from build123d import *

# Parameters (mm, degrees)
F1_DEPTH = 6.985
F2_R     = 5.08
F3_R     = 5.08
F4_R     = 1.27
F5_R     = 1.27


with BuildPart() as f1:
    # F0 (on Top) → F1 (new body)
    with BuildSketch(Plane.XY):
        with BuildLine():
            Line((13.4412104934, -0.1712630266), (10.8124273162, -2.0811858017))
            ThreePointArc((10.8124273162, -2.0811858017), (10.4719881953, -3.4025552234), (9.9707277708, -4.6716706359))
            Line((9.9707277708, -4.6716706359), (10.9748335954, -7.7619906019))
            ThreePointArc((10.9748335954, -7.7619906019), (18.0702175637, -8.5055805227), (23.2204469124, -13.442435522))
            Line((23.2204469124, -13.442435522), (27.3287873031, -8.8796612689))
            Line((27.3287873031, -8.8796612689), (26.6870015238, -2.7734774636))
            ThreePointArc((26.6870015238, -2.7734774636), (19.6185678945, -3.7402481997), (13.4412104934, -0.1712630266))
        make_face()
        with BuildLine():
            ThreePointArc((5.3205491095, 9.6401076749), (6.4720446345, 8.9080052234), (7.5241471277, 8.0391))
            Line((7.5241471277, 8.0391), (10.7735018328, 8.0391))
            ThreePointArc((10.7735018328, 8.0391), (13.6732921003, 14.5574292363), (19.960028611, 17.9300163252))
            Line((19.960028611, 17.9300163252), (16.8901194246, 23.2472550106))
            Line((16.8901194246, 23.2472550106), (10.8844708144, 24.5237950298))
            ThreePointArc((10.8844708144, 24.5237950298), (10.9792472078, 23.6942958469), (11.0109, 22.86))
            ThreePointArc((11.0109, 22.86), (9.1860721795, 16.789086006), (4.3164432849, 12.7304276409))
            Line((4.3164432849, 12.7304276409), (5.3205491095, 9.6401076749))
        make_face()
        with BuildLine():
            ThreePointArc((32.7520519625, 7.0641284914), (31.1139363339, 1.2856484198), (26.6870015238, -2.7734774636))
            Line((26.6870015238, -2.7734774636), (27.3287873031, -8.8796612689))
            Line((27.3287873031, -8.8796612689), (49.9321790072, 16.2239484353))
            Line((49.9321790072, 16.2239484353), (16.8901194246, 23.2472550106))
            Line((16.8901194246, 23.2472550106), (19.960028611, 17.9300163252))
            ThreePointArc((19.960028611, 17.9300163252), (28.869551071, 15.4561392731), (32.7520519625, 7.0641284914))
        make_face()
        with BuildLine():
            Line((3.99068165, -12.8362740124), (1.3618984728, -10.9263512372))
            ThreePointArc((1.3618984728, -10.9263512372), (0, -11.0109), (-1.3618984728, -10.9263512372))
            Line((-1.3618984728, -10.9263512372), (-3.99068165, -12.8362740124))
            ThreePointArc((-3.99068165, -12.8362740124), (-2.8242814664, -15.5589985926), (-2.4258708674, -18.4941284914))
            ThreePointArc((-2.4258708674, -18.4941284914), (-3.2526978614, -22.6803649657), (-5.6090031852, -26.2378983694))
            Line((-5.6090031852, -26.2378983694), (0, -28.7351874834))
            Line((0, -28.7351874834), (5.6090031852, -26.2378983694))
            ThreePointArc((5.6090031852, -26.2378983694), (2.5052834618, -19.8141670934), (3.99068165, -12.8362740124))
        make_face()
        with BuildLine():
            Line((27.3287873031, -8.8796612689), (23.2204469124, -13.442435522))
            ThreePointArc((23.2204469124, -13.442435522), (24.1364670634, -15.8948170204), (24.4476708674, -18.4941284914))
            ThreePointArc((24.4476708674, -18.4941284914), (17.6230073417, -28.6782014974), (5.6090031852, -26.2378983694))
            Line((5.6090031852, -26.2378983694), (0, -28.7351874834))
            Line((0, -28.7351874834), (30.8597837588, -42.4748484353))
            Line((30.8597837588, -42.4748484353), (27.3287873031, -8.8796612689))
        make_face()
        with BuildLine():
            ThreePointArc((-7.5241471277, 8.0391), (-6.4720446345, 8.9080052234), (-5.3205491095, 9.6401076749))
            Line((-5.3205491095, 9.6401076749), (-4.3164432849, 12.7304276409))
            ThreePointArc((-4.3164432849, 12.7304276409), (-9.6196583076, 17.5025665796), (-10.8844708144, 24.5237950298))
            Line((-10.8844708144, 24.5237950298), (-16.8901194246, 23.2472550106))
            Line((-16.8901194246, 23.2472550106), (-19.960028611, 17.9300163252))
            ThreePointArc((-19.960028611, 17.9300163252), (-13.6732921003, 14.5574292363), (-10.7735018328, 8.0391))
            Line((-10.7735018328, 8.0391), (-7.5241471277, 8.0391))
        make_face()
        with BuildLine():
            Line((10.8844708144, 24.5237950298), (16.8901194246, 23.2472550106))
            Line((16.8901194246, 23.2472550106), (0, 52.5018))
            Line((0, 52.5018), (-16.8901194246, 23.2472550106))
            Line((-16.8901194246, 23.2472550106), (-10.8844708144, 24.5237950298))
            ThreePointArc((-10.8844708144, 24.5237950298), (0, 33.8709), (10.8844708144, 24.5237950298))
        make_face()
        with BuildLine():
            Line((-10.9748335954, -7.7619906019), (-9.9707277708, -4.6716706359))
            ThreePointArc((-9.9707277708, -4.6716706359), (-10.4719881953, -3.4025552234), (-10.8124273162, -2.0811858017))
            Line((-10.8124273162, -2.0811858017), (-13.4412104934, -0.1712630266))
            ThreePointArc((-13.4412104934, -0.1712630266), (-19.6185678945, -3.7402481997), (-26.6870015238, -2.7734774636))
            Line((-26.6870015238, -2.7734774636), (-27.3287873031, -8.8796612689))
            Line((-27.3287873031, -8.8796612689), (-23.2204469124, -13.442435522))
            ThreePointArc((-23.2204469124, -13.442435522), (-18.0702175637, -8.5055805227), (-10.9748335954, -7.7619906019))
        make_face()
        with BuildLine():
            Line((-30.8597837588, -42.4748484353), (0, -28.7351874834))
            Line((0, -28.7351874834), (-5.6090031852, -26.2378983694))
            ThreePointArc((-5.6090031852, -26.2378983694), (-19.9088155019, -27.4021337148), (-23.2204469124, -13.442435522))
            Line((-23.2204469124, -13.442435522), (-27.3287873031, -8.8796612689))
            Line((-27.3287873031, -8.8796612689), (-30.8597837588, -42.4748484353))
        make_face()
        with BuildLine():
            Line((-19.960028611, 17.9300163252), (-16.8901194246, 23.2472550106))
            Line((-16.8901194246, 23.2472550106), (-49.9321790072, 16.2239484353))
            Line((-49.9321790072, 16.2239484353), (-27.3287873031, -8.8796612689))
            Line((-27.3287873031, -8.8796612689), (-26.6870015238, -2.7734774636))
            ThreePointArc((-26.6870015238, -2.7734774636), (-32.2131401578, 10.4666837148), (-19.960028611, 17.9300163252))
        make_face()
        with BuildLine():
            Line((-11.2691637672, 3.661573268), (-10.4719881953, 3.4025552234))
            ThreePointArc((-10.4719881953, 3.4025552234), (-9.291910918, 5.9076484579), (-7.5241471277, 8.0391))
            Line((-7.5241471277, 8.0391), (-10.7735018328, 8.0391))
            ThreePointArc((-10.7735018328, 8.0391), (-10.7410697441, 7.5520936525), (-10.7302519625, 7.0641284914))
            ThreePointArc((-10.7302519625, 7.0641284914), (-10.865814413, 5.3416442403), (-11.2691637672, 3.661573268))
        make_face()
        with BuildLine():
            ThreePointArc((-10.8124273162, -2.0811858017), (-10.9897424822, 0.6822602039), (-10.4719881953, 3.4025552234))
            Line((-10.4719881953, 3.4025552234), (-11.2691637672, 3.661573268))
            ThreePointArc((-11.2691637672, 3.661573268), (-12.1615384867, 1.6354155258), (-13.4412104934, -0.1712630266))
            Line((-13.4412104934, -0.1712630266), (-10.8124273162, -2.0811858017))
        make_face()
        with BuildLine():
            ThreePointArc((-1.3618984728, -10.9263512372), (-4.0448852036, -10.2410362025), (-6.4720446345, -8.9080052234))
            Line((-6.4720446345, -8.9080052234), (-6.9647262329, -9.586123268))
            ThreePointArc((-6.9647262329, -9.586123268), (-5.3134946628, -11.0609392356), (-3.99068165, -12.8362740124))
            Line((-3.99068165, -12.8362740124), (-1.3618984728, -10.9263512372))
        make_face()
        with BuildLine():
            Line((-6.9647262329, -9.586123268), (-6.4720446345, -8.9080052234))
            ThreePointArc((-6.4720446345, -8.9080052234), (-8.4898659458, -7.0115686571), (-9.9707277708, -4.6716706359))
            Line((-9.9707277708, -4.6716706359), (-10.9748335954, -7.7619906019))
            ThreePointArc((-10.9748335954, -7.7619906019), (-8.877618186, -8.4714519209), (-6.9647262329, -9.586123268))
        make_face()
        with BuildLine():
            Line((10.9748335954, -7.7619906019), (9.9707277708, -4.6716706359))
            ThreePointArc((9.9707277708, -4.6716706359), (8.4898659458, -7.0115686571), (6.4720446345, -8.9080052234))
            Line((6.4720446345, -8.9080052234), (6.9647262329, -9.586123268))
            ThreePointArc((6.9647262329, -9.586123268), (8.877618186, -8.4714519209), (10.9748335954, -7.7619906019))
        make_face()
        with BuildLine():
            Line((6.9647262329, -9.586123268), (6.4720446345, -8.9080052234))
            ThreePointArc((6.4720446345, -8.9080052234), (4.0448852036, -10.2410362025), (1.3618984728, -10.9263512372))
            Line((1.3618984728, -10.9263512372), (3.99068165, -12.8362740124))
            ThreePointArc((3.99068165, -12.8362740124), (5.3134946628, -11.0609392356), (6.9647262329, -9.586123268))
        make_face()
        with BuildLine():
            ThreePointArc((10.4719881953, 3.4025552234), (10.8753375495, 1.7224842511), (11.0109, 0))
            ThreePointArc((11.0109, 0), (10.9611695258, -1.0453140374), (10.8124273162, -2.0811858017))
            Line((10.8124273162, -2.0811858017), (13.4412104934, -0.1712630266))
            ThreePointArc((13.4412104934, -0.1712630266), (12.1615384867, 1.6354155258), (11.2691637672, 3.661573268))
            Line((11.2691637672, 3.661573268), (10.4719881953, 3.4025552234))
        make_face()
        with BuildLine():
            ThreePointArc((7.5241471277, 8.0391), (9.291910918, 5.9076484579), (10.4719881953, 3.4025552234))
            Line((10.4719881953, 3.4025552234), (11.2691637672, 3.661573268))
            ThreePointArc((11.2691637672, 3.661573268), (10.8001644409, 5.8252940144), (10.7735018328, 8.0391))
            Line((10.7735018328, 8.0391), (7.5241471277, 8.0391))
        make_face()
        with BuildLine():
            ThreePointArc((0, 11.0109), (2.747149178, 10.6626961977), (5.3205491095, 9.6401076749))
            Line((5.3205491095, 9.6401076749), (4.3164432849, 12.7304276409))
            ThreePointArc((4.3164432849, 12.7304276409), (2.2027494775, 12.0716816162), (0, 11.8491))
            Line((0, 11.8491), (0, 11.0109))
        make_face()
        with BuildLine():
            ThreePointArc((-5.3205491095, 9.6401076749), (-2.747149178, 10.6626961977), (0, 11.0109))
            Line((0, 11.0109), (0, 11.8491))
            ThreePointArc((0, 11.8491), (-2.2027494775, 12.0716816162), (-4.3164432849, 12.7304276409))
            Line((-4.3164432849, 12.7304276409), (-5.3205491095, 9.6401076749))
        make_face()
    extrude(amount=F1_DEPTH)

    # F2
    f2_edges = [f1.edges().sort_by_distance(p)[0] for p in [
        (-49.932179, 16.223948, 3.4925),
        (0, 52.5018, 3.4925),
        (49.932179, 16.223948, 3.4925),
        (30.859784, -42.474848, 3.4925),
        (-30.859784, -42.474848, 3.4925),
    ]]
    fillet(f2_edges, radius=F2_R)

    # F3
    f3_edges = [f1.edges().sort_by_distance(p)[0] for p in [
        (-16.890119, 23.247255, 3.4925),
        (16.890119, 23.247255, 3.4925),
        (27.328787, -8.879661, 3.4925),
        (0, -28.735187, 3.4925),
        (-27.328787, -8.879661, 3.4925),
    ]]
    fillet(f3_edges, radius=F3_R)

    # F4
    f4_edges = [f1.edges().sort_by_distance(p)[0] for p in [
        (12.443943, -34.275588, 0),
    ]]
    fillet(f4_edges, radius=F4_R)

    # F5
    f5_edges = [f1.edges().sort_by_distance(p)[0] for p in [
        (-10.079324, 35.043899, 6.985),
    ]]
    fillet(f5_edges, radius=F5_R)


solid = f1.part
Build history of the part. All positions in model axes, mm. A direction names the side the tool comes from. Round coordinates to 2 decimals unless told otherwise and drop trailing zeros. Write each loop counter-clockwise with the first axis right and the second up, starting at its lowest first coordinate (ties: lowest second). Pieces come first, ordered by that corner, then holes. Notation, with made-up numbers: M 80,-19.5 L 129,-19.5 A34 ccw 129,12.5 Z; hole C -23,-11 d8. An arc over 180 degrees is marked long. Answer as a JSON object with one key per item and string values. Group by question number.
(1) Which spindle directions (+Z, -Z, +X, -X, +Y, -Y) get a long thin tool onto all of the face, cutting with end or side? Do faces 4 (the cylindrical face through (28.356, -22.308, 0.362)), 5 (the flat face through (-28.736, -22.268, 3.461)), 6 (the cylindrical face through (12.74, -33.99, 6.62)). Say none if no direction does.
(2) Mould opens along X. For faces 1 (the cylindrical face through (-0.03, -29.216, 3.524)), 2 (the cylindrical face through (-27.777, -9.057, 3.524)), 3 (the cylindrical face through (28.36, -22.31, 6.62)) say: pulls with the +X half, pulls with the -X half, needs draft (parallel to the pull), parting line crosses it, or undercut.
(3) Cut at B-B (y = -20.5). Give the number of separate pieces and of enclosed holes in the cut face, and give its area (3 significant figures).
(4) Cut at A-A (z = 3.75). Give the cut face in (x, y), and give its area (3 significant figures).
(5) Drill centre lines: L1, parallel to Y at x = 19, z = 6.25; L2, parallel to Y at x = -14.5, z = 1; L3, parallel to X at y = -17.5, z = 4. Where is each one in solid material? Low to high.
(6) Flat gauge pins, fed straight in: pin 1 (2 mm diameter, centred on y = 10, z = 5, fed in from +X); pin 2 (2 mm diameter, centred on x = -29, z = 3, fed in from -Y). Where does each tip first touch, or does it go through?
Responses:
{
 "1": {"face 4": "-Z, +X", "face 5": "+Z, -Z, -X", "face 6": "+Z, -Y"},
 "2": {"face 1": "undercut", "face 2": "pulls with the -X half", "face 3": "pulls with the +X half"},
 "3": {"separate pieces": "3", "enclosed holes": "0", "area": "95.0 mm2"},
 "4": {"outline": "M -44.04,9.69 L -28.84,-7.2 A5.08 cw -27.57,-11.13 L -29.94,-33.72 A5.08 ccw -22.82,-38.9 L -2.07,-29.66 A5.08 cw 2.07,-29.66 L 22.82,-38.9 A5.08 ccw 29.94,-33.72 L 27.57,-11.13 A5.08 cw 28.84,-7.2 L 44.04,9.69 A5.08 ccw 41.33,18.05 L 19.1,22.78 A5.08 cw 15.76,25.21 L 4.4,44.88 A5.08 ccw -4.4,44.88 L -15.76,25.21 A5.08 cw -19.1,22.78 L -41.33,18.05 A5.08 ccw Z; hole C -21.74,7.06 d22.02; hole C -13.44,-18.49 d22.02; hole C 0,0 d22.02; hole C 0,22.86 d22.02; hole C 13.44,-18.49 d22.02; hole C 21.74,7.06 d22.02", "area": "2,060 mm2"},
 "5": {"L1": "y = -37.07 to -28, -8.99 to -3.6, 17.73 to 22.68", "L2": "y = -35.16 to -29.45, -7.53 to -1.23, 15.36 to 27.33", "L3": "x = -28.23 to -24.4, -2.47 to 2.47, 24.4 to 28.23"},
 "6": {"pin 1": "stops at x = 44.9", "pin 2": "stops at y = -38.27"}
}
